Geometry check sheet. Reference: the model listing, model coordinates, mm. Round coordinates to 2 decimals unless told otherwise and drop trailing zeros. Order: outer loops, then holes, each group sorted by start corner. A loop starts at its lowest first (then second) coordinate and runs counter-clockwise, first axis right, second up. Notation, with made-up numbers: M 50,33.25 L 95,33.25 A19 cw 95,40.25 Z; hole C 23,13 d9. An arc over 180 degrees is marked long. Answer as a JSON object with one key per item and string values. Group by question number.
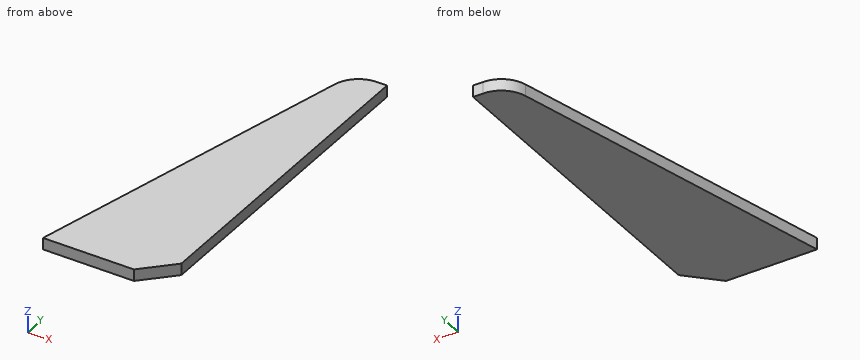
```python
from build123d import *

# Parameters (mm, degrees)
SM_BASE_FLANGE_1_DEPTH   = 6
FILLET_1_R               = 15
CUT_EXTRUDE_1_DEPTH      = 200.020099487
CUT_EXTRUDE_1_DEPTH_BACK = 200.020099487
SKETCH_4_W               = 94.166763327
SKETCH_4_H               = 540.193326504
CHAMFER_1_SIZE           = 15


# Sheet-metal steps are written as plain solids
with BuildPart() as part:
    # Sketch 2 → Базовая кромка1 (new body)
    with BuildSketch(Plane.XY):
        Polygon((-62, 0), (78, 0), (33, 183), (-17, 183), align=None)
    extrude(amount=-SM_BASE_FLANGE_1_DEPTH)

    # Скругление1
    fillet_1_edges = [part.edges().sort_by_distance(p)[0] for p in [
        (-17, 183, -3),
        (33, 183, -3),
    ]]
    fillet(fillet_1_edges, radius=FILLET_1_R)

    # Эскиз4 → Вырез-Вытянуть1 (cut, two sides: drawn at the far end of the back side and taken through both)
    with BuildSketch(Plane.XY.offset(-CUT_EXTRUDE_1_DEPTH_BACK)):
        with Locations((47.083381664, 270.096663252)):
            Rectangle(SKETCH_4_W, SKETCH_4_H)
    extrude(amount=CUT_EXTRUDE_1_DEPTH + CUT_EXTRUDE_1_DEPTH_BACK, mode=Mode.SUBTRACT)

    # Фаска1
    chamfer_1_edges = [part.edges().sort_by_distance(p)[0] for p in [
        (0, 0, -3),
    ]]
    chamfer(chamfer_1_edges, length=CHAMFER_1_SIZE)


solid = part.part
```
1) Sectioned sample at B-B (x = -23). Record the boundary of the cut face in (y, z).
2) Thickness scan on line 1 along X through (y, z) = (138, -3.2); line 2 along X through (y, z) = (95, -3.85); line 3 along Y through (x, z) = (-9.5, -5.45). Record the ranges inside material, lowest first. Write a range as [from, to].
3) Sectioned sample at C-C (y = 81). Record the boundary of the cut face in (x, z), then the cut area to 3 significant figures.
4) Sectioned sample at A-A (z = -5). Record the boundary of the cut face in (x, y), then the cut area to 3 significant figures.
Final values:
{
 "1": {"outline": "M 0,-6 L 158.6,-6 L 158.6,0 L 0,0 Z"},
 "2": {"line 1": "x = [-28.07, 0]", "line 2": "x = [-38.64, 0]", "line 3": "y = [5.5, 182.38]"},
 "3": {"outline": "M -42.08,-6 L 0,-6 L 0,0 L -42.08,0 Z", "area": "252 mm^2"},
 "4": {"outline": "M -62,0 L -15,0 L 0,15 L 0,183 L -5.24,183 A15 ccw -19.81,171.58 Z", "area": "7,090 mm^2"}
}
